Model file for the job. Use its own axes, mm. A direction names the side the tool comes from. Round coordinates to 2 decimals unless told otherwise and drop trailing zeros. Loops run counter-clockwise (first coordinate to the right, second up) from the corner with the lowest first, then second, coordinate; pieces in that order, holes last. Notation, with made-up numbers: M -12,14 L 42,14 A25 ccw 42,49 Z; hole C 36,42 d5. An arc over 180 degrees is marked long. Answer in a Markdown table with one row per item.
Autodesk Inventor part; units mm, degrees
ref_plane "YZ Plane" through (0, 0, 0) normal (1, 0, 0) x (0, 1, 0)
ref_plane "XZ Plane" through (0, 0, 0) normal (0, 1, 0) x (-1, 0, 0)
ref_plane "XY Plane" through (0, 0, 0) normal (0, 0, 1) x (1, 0, 0)
sketch "Sketch1" plane through (0, 0, 0) normal (0, 0, 1) x (1, 0, 0)
  circle A0 centre (0, 0) radius 5.15
  line L0 (-8.25, 8.25) -> (8.25, 8.25)
  line L1 (8.25, 8.25) -> (8.25, -8.25)
  line L2 (8.25, -8.25) -> (-8.25, -8.25)
  line L3 (-8.25, -8.25) -> (-8.25, 8.25)
  line L4 (-8.25, 8.25) -> (8.25, -8.25) construction
  line L5 (8.25, 8.25) -> (-8.25, -8.25) construction
  line L6 (0.75, -8.25) -> (-0.75, -8.25)
  line L7 (-0.75, -8.25) -> (-0.75, 8.25)
  line L8 (-0.75, 8.25) -> (0.75, 8.25)
  line L9 (0.75, 8.25) -> (0.75, -8.25)
  line L10 (0.75, -8.25) -> (-0.75, 8.25) construction
  line L11 (-0.75, -8.25) -> (0.75, 8.25) construction
  line L12 (8.25, 0.75) -> (-8.25, 0.75)
  line L13 (-8.25, 0.75) -> (-8.25, -0.75)
  line L14 (-8.25, -0.75) -> (8.25, -0.75)
  line L15 (8.25, -0.75) -> (8.25, 0.75)
  line L16 (8.25, 0.75) -> (-8.25, -0.75) construction
  line L17 (-8.25, 0.75) -> (8.25, -0.75) construction
  point P0 (2.2177, -5.7994)
  point P1 (6.5123, -1.5048)
  point P2 (9.7177, -1.5048)
  point P3 (9.7177, -0.0048)
  point P4 (6.5123, -0.0048)
  point P5 (2.2177, 4.2897)
  point P6 (2.2177, 7.4952)
  point P7 (0.7177, 4.2897)
  point P8 (-3.5768, -0.0048)
  point P9 (-6.7823, -0.0048)
  point P10 (-3.5768, -1.5048)
  point P11 (0.7177, -5.7994)
  point P12 (0.7177, -9.0048)
  point P13 (2.2177, -9.0048)
  point P14 (0.75, -5.0951)
  point P15 (-0.75, -5.0951)
  point P16 (5.0951, -0.75)
  point P17 (5.0951, 0.75)
  point P18 (-5.0951, -0.75)
  point P19 (-5.0951, 0.75)
  point P20 (0.75, 5.0951)
  point P21 (-0.75, 5.0951)
  dimension "d0" = 10.3
  dimension "d1" = 16.5
  dimension "d2" = 1.5
  dimension "d3" = 1.5
  dimension "d4" = 16.5
extrude "face" add sketch "Sketch1" against normal blind 10 contours A0 L12 L1 L14 | A0 L9 L0 L1 L12 | L14 L1 L2 L9 A0 | A0 L7 L0 L9 | L9 L2 L7 A0 | A0 L12 L3 L0 L7 | L7 L2 L3 L14 A0 | A0 L14 L3 L12
extrude "Extrusion2" cut sketch "Sketch1" against normal blind 7 contours A0 L12 L1 L14 | A0 L7 L0 L9 | L9 L2 L7 A0 | A0 L14 L3 L12
fillet "Fillet1" radius 6 4 edges at (-8.25, 8.25, -5) (8.25, -8.25, -5) (8.25, 8.25, -5) (-8.25, -8.25, -5)
fillet "Fillet2" radius 2 8 edges at (-8.25, 0, -10) (-6.4926, -6.4926, -10) (0, -8.25, -10) (6.4926, -6.4926, -10) (8.25, 0, -10) (6.4926, 6.4926, -10) (0, 8.25, -10) (-6.4926, 6.4926, -10)
fillet "Fillet4" radius 2 8 edges at (0.75, -6.6725, 0) (-0.75, -6.6725, 0) (-6.6725, -0.75, 0) (-6.6725, 0.75, 0) (-0.75, 6.6725, 0) (0.75, 6.6725, 0) (6.6725, 0.75, 0) (6.6725, -0.75, 0)
sketch "Sketch6" plane through (0, 0, -10) normal (0, 0, -1) x (-1, 0, 0)
  circle A0 centre (0, 0) radius 5.15
  line L0 (6.25, 2.25) -> (6.25, -2.25)
  arc A1 (6.25, 2.25) -> (2.25, 6.25) centre (2.25, 2.25) ccw
  line L1 (-2.25, 6.25) -> (2.25, 6.25)
  arc A2 (-2.25, 6.25) -> (-6.25, 2.25) centre (-2.25, 2.25) ccw
  line L2 (-6.25, -2.25) -> (-6.25, 2.25)
  arc A3 (-6.25, -2.25) -> (-2.25, -6.25) centre (-2.25, -2.25) ccw
  line L3 (2.25, -6.25) -> (-2.25, -6.25)
  arc A4 (2.25, -6.25) -> (6.25, -2.25) centre (2.25, -2.25) ccw
extrude "Extrusion9" add sketch "Sketch6" along normal blind 7 contours A0 | L0 A4 L3 A3 L2 A2 L1 A1
sketch "Sketch7" plane through (0, 0, -17) normal (0, 0, -1) x (-1, 0, 0)
  line L0 (4.5207, 0) -> (2.2603, -3.915)
  line L1 (2.2603, -3.915) -> (-2.2603, -3.915)
  line L2 (-2.2603, -3.915) -> (-4.5207, 0)
  line L3 (-4.5207, 0) -> (-2.2603, 3.915)
  line L4 (-2.2603, 3.915) -> (2.2603, 3.915)
  line L5 (2.2603, 3.915) -> (4.5207, 0)
  line L6 (2.3758, -4.115) -> (4.7516, 0)
  line L7 (4.7516, 0) -> (2.3758, 4.115)
  line L8 (2.3758, 4.115) -> (-2.3758, 4.115)
  line L9 (-2.3758, 4.115) -> (-4.7516, 0)
  line L10 (-4.7516, 0) -> (-2.3758, -4.115)
  line L11 (-2.3758, -4.115) -> (2.3758, -4.115)
  circle A0 centre (0, 0) radius 3.5
  dimension "d34" = 7.83
  dimension "d35" = 0.2
  dimension "d38" = 7
extrude "Extrusion10" cut sketch "Sketch7" against normal blind 3.5 contours L0 L1 L2 L3 L4 L5 | L11 L10 L9 L8 L7 L6 | A0
sketch "Sketch8" plane through (0, 0, -10) normal (0, 0, 1) x (1, 0, 0)
  line L0 (4.5207, 0) -> (2.2603, -3.915)
  line L1 (2.2603, -3.915) -> (-2.2603, -3.915)
  line L2 (-2.2603, -3.915) -> (-4.5207, 0)
  line L3 (-4.5207, 0) -> (-2.2603, 3.915)
  line L4 (-2.2603, 3.915) -> (2.2603, 3.915)
  line L5 (2.2603, 3.915) -> (4.5207, 0)
  line L6 (2.4335, -4.215) -> (4.8671, 0)
  line L7 (4.8671, 0) -> (2.4335, 4.215)
  line L8 (2.4335, 4.215) -> (-2.4335, 4.215)
  line L9 (-2.4335, 4.215) -> (-4.8671, 0)
  line L10 (-4.8671, 0) -> (-2.4335, -4.215)
  line L11 (-2.4335, -4.215) -> (2.4335, -4.215)
  circle A0 centre (0, 0) radius 3.5
  dimension "d41" = 7.83
  dimension "d42" = 0.3
  dimension "d43" = 7
extrude "Extrusion12" [suppressed]
sketch "Sketch9" plane through (0, 0, -17) normal (0, 0, -1) x (-1, 0, 0)
  circle A0 centre (0, 0) radius 2.6
  circle A1 centre (0, 0) radius 4
  dimension "d46" = 5.2
  dimension "d47" = 8
extrude "Extrusion13" [suppressed]
extrude "Extrusion14" [suppressed]
properties part number "adapter-02"
1. Wall check: probe 1 along Y at (x, z) = (0.25, -13.75) (3 decimals); probe 2 along Y at (x, z) = (-7.5, -6); probe 3 along Z at (x, y) = (2.75, -1.5). Give the ranges that are in metal, low to high.
Verdict:
| item | result |
|---|---|
| probe 1 | y = -6.25 to -4.115, 4.115 to 6.25 |
| probe 2 | y = -5.15 to -0.75, 0.75 to 5.15 |
| probe 3 | z = -13.5 to -10 |
2. Saw through at B-B (z = -16). Write the cut outline in (x, y) (3 decimals), and give its area (3 significant figures).
Verdict:
| item | result |
|---|---|
| outline | M -6.25,-2.25 A4 ccw -2.25,-6.25 L 2.25,-6.25 A4 ccw 6.25,-2.25 L 6.25,2.25 A4 ccw 2.25,6.25 L -2.25,6.25 A4 ccw -6.25,2.25 Z; hole M -4.752,0 L -2.376,-4.115 L 2.376,-4.115 L 4.752,0 L 2.376,4.115 L -2.376,4.115 Z |
| area | 83.9 mm² |
3. Saw through at C-C (x = 0). Write the cut outline in (y, z) (3 decimals), and give its area (3 significant figures).
Verdict:
| item | result |
|---|---|
| outline | M -8.25,-8 A2 ccw -6.25,-10 L -6.25,-17 L -4.115,-17 L -4.115,-13.5 L 4.115,-13.5 L 4.115,-17 L 6.25,-17 L 6.25,-10 A2 ccw 8.25,-8 L 8.25,-7 L 5.15,-7 L 5.15,-10 L -5.15,-10 L -5.15,-7 L -8.25,-7 Z |
| area | 75.6 mm² |
4. Saw through at A-A (z = -6.5). Write the cut outline in (x, y), and give its area (3 significant figures).
Verdict:
| item | result |
|---|---|
| outline | M -8.25,-2.25 A6 ccw -2.25,-8.25 L -0.75,-8.25 L -0.75,-5.1 A5.15 cw -5.1,-0.75 L -8.25,-0.75 Z; M -8.25,0.75 L -5.1,0.75 A5.15 cw -0.75,5.1 L -0.75,8.25 L -2.25,8.25 A6 ccw -8.25,2.25 Z; M 0.75,-8.25 L 2.25,-8.25 A6 ccw 8.25,-2.25 L 8.25,-0.75 L 5.1,-0.75 A5.15 cw 0.75,-5.1 Z; M 0.75,5.1 A5.15 cw 5.1,0.75 L 8.25,0.75 L 8.25,2.25 A6 ccw 2.25,8.25 L 0.75,8.25 Z |
| area | 139 mm² |
5. Saw through at D-D (z = -12.75). Write the cut outline in (x, y).
Verdict:
| item | result |
|---|---|
| outline | M -6.25,-2.25 A4 ccw -2.25,-6.25 L 2.25,-6.25 A4 ccw 6.25,-2.25 L 6.25,2.25 A4 ccw 2.25,6.25 L -2.25,6.25 A4 ccw -6.25,2.25 Z |
6. Pin check, flat tips, straight feed: pin 1 (2.5 mm diameter, centred on x = 6.5, z = -5, fed in from +Y); pin 2 (0.8 mm diameter, centred on x = -6, y = 0, fed in from +Z); pin 3 (3 mm diameter, centred on y = -6, z = -14, fed in from +X). Stop position of each tip, or through.
Verdict:
| item | result |
|---|---|
| pin 1 | stops at y = 7.45 |
| pin 2 | stops at z = -7 |
| pin 3 | stops at x = 5.56 |
7. Tool access for faces 1 (the cylindrical face through (5.109, 5.047, -13.451)), 2 (the cylindrical face through (5.047, -5.109, -13.451)), 3 (the flat face through (0.75, 7, -4)), 4 (the flat face through (0, -4.115, -15)): list every direction of +Z, -Z, +X, -X, +Y, -Y with a clear straight run to the whole face (end or side of a thin tool).
Verdict:
| item | result |
|---|---|
| face 1 | -Z, +X, +Y |
| face 2 | -Z, +X, -Y |
| face 3 | +Z, +Y, -Y |
| face 4 | -Z |
8. Mould opens along Y. For faces 5 (the flat face through (6.25, 0, -13)), 6 (the flat face through (7, -0.75, -4)), 7 (the cylindrical face through (-6.539, 6.446, -4.056)) say: +Y half, -Y half, draft (parallel to the pull), parting line (faces both ways), or undercut.
Verdict:
| item | result |
|---|---|
| face 5 | draft |
| face 6 | undercut |
| face 7 | +Y half |
